from build123d import *

# Parameters (mm, degrees)
SKETCH1_R           = 12.5
BOSS_EXTRUDE1_DEPTH = 67
SKETCH2_R           = 3.5
BOSS_EXTRUDE2_DEPTH = 2.5
BOSS_EXTRUDE3_DEPTH = 10
SKETCH4_R           = 1.5
CUT_EXTRUDE1_DEPTH  = 12.7


with BuildPart() as part:
    # Sketch1 → Boss-Extrude1 (new body)
    with BuildSketch(Plane.XY):
        Circle(SKETCH1_R)
    extrude(amount=BOSS_EXTRUDE1_DEPTH)

    # Sketch2 → Boss-Extrude2 (add)
    with BuildSketch(Plane(origin=(0, 0, 0), x_dir=(-1, 0, 0), z_dir=(0, 0, -1))):
        Circle(SKETCH2_R)
    extrude(amount=BOSS_EXTRUDE2_DEPTH)

    # Sketch3 → Boss-Extrude3 (add)
    with BuildSketch(Plane(origin=(0, 0, -2.5), x_dir=(-1, 0, 0), z_dir=(0, 0, -1))):
        with BuildLine():
            Line((-1.322875656, 1.5), (1.322875656, 1.5))
            ThreePointArc((1.322875656, 1.5), (0, -2), (-1.322875656, 1.5))
        make_face()
    extrude(amount=BOSS_EXTRUDE3_DEPTH)

    # Sketch4 → Cut-Extrude1 (cut)
    with BuildSketch(Plane(origin=(0, 0, 0), x_dir=(-1, 0, 0), z_dir=(0, 0, -1))):
        with Locations((0, 8.5)):
            Circle(SKETCH4_R)
    cut_extrude1 = extrude(amount=-CUT_EXTRUDE1_DEPTH, mode=Mode.SUBTRACT)

    # Mirror1: Cut-Extrude1 across plane
    add(cut_extrude1.mirror(Plane.ZX), mode=Mode.SUBTRACT)


solid = part.part
For this review, take the finished solid that the model builds, in its own axes (mm). A direction names the side the tool comes from. Coordinates: 2 decimals unless noted, no trailing zeros. Order: outer loops, then holes, each group sorted by start corner. A loop starts at its lowest first (then second) coordinate and runs counter-clockwise, first axis right, second up. Notation, with made-up numbers: (37, 65.25) - (44, 65.25) arc R8 ccw to (44, 79.25) - close; hole circle Ø11 at (77, 70). An arc over 180 degrees is marked (long way). Answer as CSV lines item,"result". Start each with the question number.
1) Machinability: for faces 4 (the flat face through (0, 1.5, -7)), 5 (the cylindrical face through (0, -7, 6)), 6 (the flat face through (0, 0, 67)), which of the approach directions +Z, -Z, +X, -X, +Y, -Y give a long, thin tool a straight path to every point of the face, cutting with its end or side? Answer none if there is none.
2) Add section D-D (z = -4). State the section outline as (x, y) points.
3) Add section A-A (x = 0). State the section outline as (y, z) points.
4) Add section B-B (y = 0). State the section outline as (x, z) points, then the cut area to 3 significant figures.
5) To check wall thickness, follow line 1 along Y through (x, z) = (0, 4.25); line 2 along Z through (x, y) = (-9.75, -7); line 3 along X through (y, z) = (-8.5, 5). State the ranges of each line that lie inside material, in increasing order. Write a range as [from, to].
6) Draft analysis for pull direction Y (two halves, no side actions). For faces 1 (the cylindrical face through (-3.233, -1.341, -1.232)), 2 (the flat face through (3, -3, 0)), 3 (the flat face through (0, -9, 12.7)), state which applies: +Y half, -Y half, draft (parallel to the pull), parting line (faces both ways), or undercut.
7) Add section C-C (z = 5). State the section outline as (x, y) points.
8) Insertion check: P1, Ø1.5, axis at y = -4, z = 50, coming from the +X side; P2, Ø3, axis at x = -0.5, z = -7, coming from the +Y side; P3, Ø1.5, axis at x = 4, y = -2, coming from the -Z side; P4, Ø1.5, axis at x = 9.5, y = -10, coming from the +Z side. Each pin has a flat end and moves straight along its axis. Give the tip position at first contact, or say it passes through.
Result:
1,face 4,"-Z, +X, -X, +Y"
1,face 5,"-Z"
1,face 6,"+Z, +X, -X, +Y, -Y"
2,outline,"(-1.32, 1.5) arc R2 ccw (long way) to (1.32, 1.5) - close"
3,outline,"(-12.5, 0) - (-10, 0) - (-10, 12.7) - (-7, 12.7) - (-7, 0) - (-3.5, 0) - (-3.5, -2.5) - (-2, -2.5) - (-2, -12.5) - (1.5, -12.5) - (1.5, -2.5) - (3.5, -2.5) - (3.5, 0) - (7, 0) - (7, 12.7) - (10, 12.7) - (10, 0) - (12.5, 0) - (12.5, 67) - (-12.5, 67) - close"
4,outline,"(-12.5, 0) - (-3.5, 0) - (-3.5, -2.5) - (-2, -2.5) - (-2, -12.5) - (2, -12.5) - (2, -2.5) - (3.5, -2.5) - (3.5, 0) - (12.5, 0) - (12.5, 67) - (-12.5, 67) - close"
4,area,"1,730 mm^2"
5,line 1,"[-12.5, -10], [-7, 7], [10, 12.5]"
5,line 2,"[0, 67]"
5,line 3,"[-9.17, -1.5], [1.5, 9.17]"
6,face 1,"parting line"
6,face 2,"draft"
6,face 3,"undercut"
7,outline,"circle Ø25 at (0, 0); hole circle Ø3 at (0, -8.5); hole circle Ø3 at (0, 8.5)"
8,P1,"x = 12.07"
8,P2,"y = 1.5"
8,P3,"z = 0"
8,P4,"through"
